```python
from build123d import *

# Parameters (mm, degrees)
SKETCH1_W            = 18.25
SKETCH1_H            = 40
OUTLINE_DEPTH        = 40
OUTLINE_DEPTH_BACK   = 40
SKETCH2_W            = 40
SKETCH2_H            = 80
EXTRUSION15_DEPTH    = 6
CAMERA_MOUNT_D       = 24.5364
SKETCH5_R            = 17.5
SKETCH5_R_2          = 12.268
EXTRUSION19_DEPTH    = 5.9562
SKETCH10_W           = 80
SKETCH10_H           = 80
SKETCH10_R           = 17.5
CUT_EXTRUDE1_DEPTH   = 3
SKETCH6_W            = 80
SKETCH6_H            = 40
EXTRUSION21_DEPTH    = 6
SKETCH7_W            = 50
SKETCH7_H            = 50
EXTRUSION22_DEPTH    = 9
FILLET4_R            = 3.175
HOLE7_D              = 3.3
HOLE7_DEPTH          = 12
HOLE7_TIP            = 0.991420021
SKETCH11_OUTSIDE_W   = 105.14
SKETCH11_OUTSIDE_H   = 105.14
SKETCH11_OUTSIDE_W_2 = 74
SKETCH11_OUTSIDE_H_2 = 74
CUT_EXTRUDE2_DEPTH   = 16.25
CUT_EXTRUDE3_DEPTH   = 3


with BuildPart() as part:
    # Sketch1 → Outline (new body, two sides)
    with BuildSketch(Plane.YZ) as outline_sk:
        Polygon((18.25, 40), (5.33, 40), (0, 40), (0, 0), (18.25, 0), align=None)
        with Locations((9.125, -20)):
            Rectangle(SKETCH1_W, SKETCH1_H)
    extrude(amount=OUTLINE_DEPTH)
    extrude(outline_sk.sketch, amount=-OUTLINE_DEPTH_BACK)

    # Sketch2 → Extrusion15 (cut)
    with BuildSketch(Plane.XZ):
        Rectangle(SKETCH2_W, SKETCH2_H)
    extrude(amount=-EXTRUSION15_DEPTH, mode=Mode.SUBTRACT)

    # Camera mount (through all)
    with Locations(Plane(origin=(0, 18.25, 0), x_dir=(1, 0, 0), z_dir=(0, 1, 0))):
        with Locations((0, 0)):
            Hole(CAMERA_MOUNT_D / 2)

    # Sketch5 → Extrusion19 (add)
    with BuildSketch(Plane(origin=(0, 18.25, 0), x_dir=(-1, 0, 0), z_dir=(0, 1, 0))):
        Circle(SKETCH5_R)
        Circle(SKETCH5_R_2, mode=Mode.SUBTRACT)
    extrude(amount=EXTRUSION19_DEPTH)

    # Sketch10 → Cut-Extrude1 (cut)
    with BuildSketch(Plane(origin=(0, 18.25, 0), x_dir=(1, 0, 0), z_dir=(0, 1, 0))):
        Rectangle(SKETCH10_W, SKETCH10_H)
        Circle(SKETCH10_R, mode=Mode.SUBTRACT)
    extrude(amount=-CUT_EXTRUDE1_DEPTH, mode=Mode.SUBTRACT)

    # Sketch6 → Extrusion21 (cut)
    with BuildSketch(Plane.XZ):
        Rectangle(SKETCH6_W, SKETCH6_H)
    extrude(amount=-EXTRUSION21_DEPTH, mode=Mode.SUBTRACT)

    # Sketch7 → Extrusion22 (cut)
    with BuildSketch(Plane.XZ):
        Rectangle(SKETCH7_W, SKETCH7_H)
    extrude(amount=-EXTRUSION22_DEPTH, mode=Mode.SUBTRACT)

    # Fillet4
    fillet4_edges = [part.edges().sort_by_distance(p)[0] for p in [
        (-25, 4.5, 25),
        (25, 4.5, -25),
        (25, 4.5, 25),
        (-25, 4.5, -25),
        (-17.5, 15.25, 0),
    ]]
    fillet(fillet4_edges, radius=FILLET4_R)

    # Hole7
    with Locations(Plane(origin=(0, 0, 0), x_dir=(-1, 0, 0), z_dir=(0, -1, 0))):
        with Locations((27.5, 27.5), (-27.5, 27.5), (-27.5, -27.5), (27.5, -27.5)):
            Hole(HOLE7_D / 2, depth=HOLE7_DEPTH)
            with Locations((0, 0, -(HOLE7_DEPTH + HOLE7_TIP / 2))):  # 118° drill point
                Cone(0, HOLE7_D / 2, HOLE7_TIP, mode=Mode.SUBTRACT)

    # Sketch11 outside → Cut-Extrude2 (cut, through all)
    with BuildSketch(Plane(origin=(0, 15.25, 0), x_dir=(1, 0, 0), z_dir=(0, 1, 0))):
        Rectangle(SKETCH11_OUTSIDE_W, SKETCH11_OUTSIDE_H)
        Rectangle(SKETCH11_OUTSIDE_W_2, SKETCH11_OUTSIDE_H_2, mode=Mode.SUBTRACT)
    extrude(amount=-CUT_EXTRUDE2_DEPTH, mode=Mode.SUBTRACT)

    # Sketch13 → Cut-Extrude3 (cut)
    with BuildSketch(Plane.XZ.offset(-9)):
        with BuildLine():
            Line((21.825, 25), (-21.825, 25))
            ThreePointArc((-21.825, 25), (-24.07006403, 24.07006403), (-25, 21.825))
            Line((-25, 21.825), (-25, -21.825))
            ThreePointArc((-25, -21.825), (-24.07006403, -24.07006403), (-21.825, -25))
            Line((-21.825, -25), (21.825, -25))
            ThreePointArc((21.825, -25), (24.07006403, -24.07006403), (25, -21.825))
            Line((25, -21.825), (25, 21.825))
            ThreePointArc((25, 21.825), (24.07006403, 24.07006403), (21.825, 25))
        make_face()
    extrude(amount=-CUT_EXTRUDE3_DEPTH, mode=Mode.SUBTRACT)


solid = part.part
```
The listing builds one solid part. Answer for the finished solid, in the listing's coordinates (mm). A direction names the side the tool comes from. Round coordinates to 2 decimals unless told otherwise and drop trailing zeros. Loops run counter-clockwise (first coordinate to the right, second up) from the corner with the lowest first, then second, coordinate; pieces in that order, holes last. Notation, with made-up numbers: (40, -12.75) - (66, -12.75) arc R14 ccw to (66, 2.25) - close; hole circle Ø1 at (64.5, 43). An arc over 180 degrees is marked (long way). Return JSON: item names as keys, results as strings. Group by question number.
1. Each of these flat-tipped pins is pushed along its axis until it touches: P1, Ø19.5, axis at x = -6, z = -0.5, coming from the -Y side; P2, Ø6, axis at x = 6, z = 29.5, coming from the -Y side; P3, Ø1, axis at y = 21, z = 7, coming from the -X side. Where does it stop, or does it pass through?
2. Consider probe 1 along Z at (x, y) = (-27.5, 4.25); probe 2 along Z at (x, y) = (27.5, 7.75). Determine where each line is inside the solid, lowest interval first.
3. Which of the six approach directions +Z, -Z, +X, -X, +Y, -Y give full straight-line access (tool end or side, diameter ignored) to faces 1 (the flat face through (0, 9, 25)), 2 (the flat face through (-31, 3, 20)), 3 (the flat face through (20, 3, 31)), 4 (the flat face through (-17, 15.25, -17))?
4. The part is cut by section A-A on y = 7.75. Determine the outline of the cut face in (x, z) (3 decimals).
Resolved:
{
 "1": {"P1": "stops at y = 12", "P2": "stops at y = 6", "P3": "stops at x = -16.25"},
 "2": {"probe 1": "z = -37 to -29.15, -25.85 to -20, 20 to 25.85, 29.15 to 37", "probe 2": "z = -37 to -29.15, -25.85 to 25.85, 29.15 to 37"},
 "3": {"face 1": "-Y", "face 2": "+X, -X, -Y", "face 3": "+Z, -Z, -Y", "face 4": "+Y"},
 "4": {"outline": "(-37, -37) - (37, -37) - (37, 37) - (-37, 37) - close; hole circle Ø3.3 at (-27.5, -27.5); hole circle Ø3.3 at (-27.5, 27.5); hole (-25, -21.825) arc R3.175 ccw to (-21.825, -25) - (21.825, -25) arc R3.175 ccw to (25, -21.825) - (25, 21.825) arc R3.175 ccw to (21.825, 25) - (-21.825, 25) arc R3.175 ccw to (-25, 21.825) - close; hole circle Ø3.3 at (27.5, -27.5); hole circle Ø3.3 at (27.5, 27.5)"}
}
